The listing builds one solid part. Answer for the finished solid, in the listing's coordinates (mm). Face numbers are marked on the shaded views. A direction names the side the tool comes from. Give positions to 0.01 mm unless a question says otherwise; leave off trailing zeros. Write each loop counter-clockwise with the first axis right and the second up, starting at its lowest first coordinate (ties: lowest second). Pieces come first, ordered by that corner, then holes. Notation, with made-up numbers: M -34,-27.75 L 15,-27.75 A31 ccw 15,4.25 Z; hole C 62.25,-12.5 d11. An arc over 180 degrees is marked long. Answer as a JSON object with one key per item and string values.
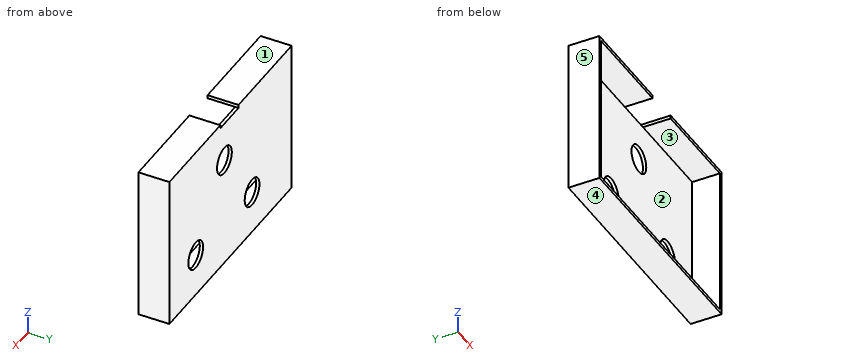
```python
from build123d import *

# Parameters (mm, degrees)
SKETCH1_W           = 235.712
SKETCH1_H           = 159.512
BOSS_EXTRUDE1_DEPTH = 31.75
SKETCH2_W           = 228.9048
SKETCH2_H           = 152.7048
CUT_EXTRUDE1_DEPTH  = 28.3464
SKETCH3_W           = 35.052
SKETCH3_H           = 3.4036
CUT_EXTRUDE2_DEPTH  = 287.377875521
SKETCH4_R           = 14.224
CUT_EXTRUDE3_DEPTH  = 287.377875521


with BuildPart() as part:
    # Sketch1 → Boss-Extrude1 (new body)
    with BuildSketch(Plane(origin=(0, 0, 0), x_dir=(1, 0, 0), z_dir=(0, 1, 0))):
        with Locations((117.856, 79.756)):
            Rectangle(SKETCH1_W, SKETCH1_H)
    extrude(amount=BOSS_EXTRUDE1_DEPTH)

    # Sketch2 → Cut-Extrude1 (cut)
    with BuildSketch(Plane.XZ):
        with Locations((117.856, -79.756)):
            Rectangle(SKETCH2_W, SKETCH2_H)
    extrude(amount=-CUT_EXTRUDE1_DEPTH, mode=Mode.SUBTRACT)

    # Sketch3 → Cut-Extrude2 (cut, through all)
    with BuildSketch(Plane(origin=(0, 31.75, 0), x_dir=(1, 0, 0), z_dir=(0, 1, 0))):
        with Locations((119.888, 1.7018)):
            Rectangle(SKETCH3_W, SKETCH3_H)
    extrude(amount=-CUT_EXTRUDE2_DEPTH, mode=Mode.SUBTRACT)

    # Sketch4 → Cut-Extrude3 (cut, through all)
    with BuildSketch(Plane(origin=(0, 31.75, 0), x_dir=(1, 0, 0), z_dir=(0, 1, 0))):
        with Locations(Location((76.2, 115.062, 0), (0, 0, 270))):
            Circle(SKETCH4_R)
        with Locations(Location((129.54, 44.45, 0), (0, 0, 270))):
            Circle(SKETCH4_R)
        with Locations(Location((184.912, 115.062, 0), (0, 0, 270))):
            Circle(SKETCH4_R)
    extrude(amount=-CUT_EXTRUDE3_DEPTH, mode=Mode.SUBTRACT)


solid = part.part
```
1. The mould has two halves that part along X. Classify the marked faces 3, 4 and 5: released by +X, released by -X, zero draft, split by the parting line, or undercut.
Verdict:
{"face 3": "undercut", "face 4": "zero draft", "face 5": "released by -X"}
2. For the marked faces 1 and 2, determine the directions among +Z, -Z, +X, -X, +Y, -Y from which every point of the face is accessible in a straight line to the end or side of a thin tool.
Verdict:
{"face 1": "+Z, +X, -X, +Y, -Y", "face 2": "-Y"}
3. Flat-ended cylindrical pins translate along their axes: pin 1 (1.7 mm diameter, centred on x = 119, y = 31, fed in from +Z); pin 2 (1 mm diameter, centred on x = 208, z = -77.5, fed in from -Y). Find the tip coordinate at first contact, or state that the pin passes through.
Verdict:
{"pin 1": "stops at z = -3.4", "pin 2": "stops at y = 28.35"}
4. A cutting plane is placed at C-C, the plane x = 99. Give the vertices of the cut face in (y, z), plus the area to 3 significant figures.
Verdict:
{"outline": "M 0,-159.51 L 31.75,-159.51 L 31.75,0 L 0,0 L 0,-3.4 L 28.35,-3.4 L 28.35,-156.11 L 0,-156.11 Z", "area": "736 mm2"}
5. A cutting plane is placed at A-A, the plane x = 129.54. Give the vertices of the cut face in (y, z).
Verdict:
{"outline": "M 0,-159.51 L 31.75,-159.51 L 31.75,-58.67 L 28.35,-58.67 L 28.35,-156.11 L 0,-156.11 Z; M 28.35,-30.23 L 31.75,-30.23 L 31.75,-3.4 L 28.35,-3.4 Z"}
6. A cutting plane is placed at D-D, the plane y = 6. Give the vertices of the cut face in (x, z).
Verdict:
{"outline": "M 0,-159.51 L 235.71,-159.51 L 235.71,0 L 137.41,0 L 137.41,-3.4 L 232.31,-3.4 L 232.31,-156.11 L 3.4,-156.11 L 3.4,-3.4 L 102.36,-3.4 L 102.36,0 L 0,0 Z"}
7. A cutting plane is placed at B-B, the plane z = -44.45. Give the vertices of the cut face in (x, y).
Verdict:
{"outline": "M 0,0 L 3.4,0 L 3.4,28.35 L 115.32,28.35 L 115.32,31.75 L 0,31.75 Z; M 143.76,28.35 L 232.31,28.35 L 232.31,0 L 235.71,0 L 235.71,31.75 L 143.76,31.75 Z"}
8. Consider line 1 along Z through (x, y) = (64, 7); line 2 along X through (y, z) = (26, -75); line 3 along Z through (x, y) = (76, 29). Determine where each line is inside the solid, lowest interval first.
Verdict:
{"line 1": "z = -159.51 to -156.11, -3.4 to 0", "line 2": "x = 0 to 3.4, 232.31 to 235.71", "line 3": "z = -159.51 to -129.28, -100.84 to 0"}
